```python
from build123d import *

# Parameters (mm, degrees)
BOSS_EXTRUDE1_DEPTH = 10


with BuildPart() as part:
    # Sketch1 → Boss-Extrude1 (new body)
    with BuildSketch(Plane.XY):
        with BuildLine():
            Line((138.578606851, 12), (138.578606851, 0))
            Line((138.578606851, 0), (37.275, 0))
            Line((37.275, 0), (37.275, 12))
            Line((37.275, 12), (38.178606851, 12))
            ThreePointArc((38.178606851, 12), (39.211044436, 12.32552632), (39.870053568, 13.184363742))
            Line((39.870053568, 13.184363742), (44.171321406, 25.002))
            Line((44.171321406, 25.002), (49.228678594, 25.002))
            Line((49.228678594, 25.002), (53.529946432, 13.184363742))
            ThreePointArc((53.529946432, 13.184363742), (54.188955564, 12.32552632), (55.221393149, 12))
            Line((55.221393149, 12), (57.028606851, 12))
            ThreePointArc((57.028606851, 12), (58.061044436, 12.32552632), (58.720053568, 13.184363742))
            Line((58.720053568, 13.184363742), (63.021321406, 25.002))
            Line((63.021321406, 25.002), (68.078678594, 25.002))
            Line((68.078678594, 25.002), (72.379946432, 13.184363742))
            ThreePointArc((72.379946432, 13.184363742), (73.038955564, 12.32552632), (74.071393149, 12))
            Line((74.071393149, 12), (75.878606851, 12))
            ThreePointArc((75.878606851, 12), (76.911044436, 12.32552632), (77.570053568, 13.184363742))
            Line((77.570053568, 13.184363742), (81.871321406, 25.002))
            Line((81.871321406, 25.002), (86.928678594, 25.002))
            Line((86.928678594, 25.002), (91.229946432, 13.184363742))
            ThreePointArc((91.229946432, 13.184363742), (91.888955564, 12.32552632), (92.921393149, 12))
            Line((92.921393149, 12), (94.728606851, 12))
            ThreePointArc((94.728606851, 12), (95.761044436, 12.32552632), (96.420053568, 13.184363742))
            Line((96.420053568, 13.184363742), (100.721321406, 25.002))
            Line((100.721321406, 25.002), (105.778678594, 25.002))
            Line((105.778678594, 25.002), (110.079946432, 13.184363742))
            ThreePointArc((110.079946432, 13.184363742), (110.738955564, 12.32552632), (111.771393149, 12))
            Line((111.771393149, 12), (113.578606851, 12))
            Line((113.578606851, 12), (138.578606851, 12))
        make_face()
    extrude(amount=BOSS_EXTRUDE1_DEPTH)


solid = part.part
```
The listing builds one solid part. Answer for the finished solid, in the listing's coordinates (mm). A direction names the side the tool comes from. Coordinates: 2 decimals unless noted, no trailing zeros. Write each loop counter-clockwise with the first axis right and the second up, starting at its lowest first coordinate (ties: lowest second). Pieces come first, ordered by that corner, then holes.
Q1. Section C-C, the plane x = 131 is taken. Write down the section's boundary in (y, z), then the cut area to 3 significant figures.
Returned:
outline: (0, 0) - (12, 0) - (12, 10) - (0, 10) - close
area: 120 mm2
Q2. Given P1, Ø0.5, axis at x = 37.5, z = 6.5, coming from the +Y side; P2, Ø2, axis at x = 56.5, z = 4.5, coming from the +Y side; P3, Ø1.5, axis at x = 108.5, y = 16, coming from the -Z side, each flat-ended and moving along its own axis, determine where each tip first touches the part or whether it passes through.
Returned:
P1: stops at y = 12
P2: stops at y = 12.06
P3: stops at z = 0
Q3. Which of the six approach directions +Z, -Z, +X, -X, +Y, -Y give full straight-line access (tool end or side, diameter ignored) to faces 1 (the cylindrical face through (54.18, 12.33, 4.93)), 2 (the flat face through (41.99, 19.01, 4.93)), 3 (the flat face through (125, 12, 5))?
Returned:
face 1: +Z, -Z, +Y
face 2: +Z, -Z, -X, +Y
face 3: +Z, -Z, +X, +Y
Q4. Section B-B, the plane y = 19 is taken. Write down the section's boundary in (x, z).
Returned:
outline: (41.99, 0) - (51.41, 0) - (51.41, 10) - (41.99, 10) - close; (60.84, 0) - (70.26, 0) - (70.26, 10) - (60.84, 10) - close; (79.69, 0) - (89.11, 0) - (89.11, 10) - (79.69, 10) - close; (98.54, 0) - (107.96, 0) - (107.96, 10) - (98.54, 10) - close
Q5. The mould has two halves that part along X. Classify faces 4 (the cylindrical face through (76.9, 12.32, 4.93)), 5 (the flat face through (37.275, 6, 5)), 6 (the flat face through (107.899, 19.176, 4.93)), 7 (the flat face through (103, 25.002, 5)): released by +X, released by -X, zero draft, split by the parting line, or undercut.
Returned:
face 4: undercut
face 5: released by -X
face 6: released by +X
face 7: zero draft
Q6. Section D-D, the plane x = 107.5 is taken. Write down the section's boundary in (y, z), then the cut area to 3 significant figures.
Returned:
outline: (0, 0) - (20.27, 0) - (20.27, 10) - (0, 10) - close
area: 203 mm2
Q7. Find the intervals of material crossed by line 1 along X through (y, z) = (23.25, 3.5); line 2 along X through (y, z) = (20, 0.75); line 3 along Y through (x, z) = (120.5, 9), in increasing order.
Returned:
line 1: x = 43.53 to 49.87, 62.38 to 68.72, 81.23 to 87.57, 100.08 to 106.42
line 2: x = 42.35 to 51.05, 61.2 to 69.9, 80.05 to 88.75, 98.9 to 107.6
line 3: y = 0 to 12
Q8. Section A-A, the plane z = 2.5 is taken. Write down the section's boundary in (x, y) (3 decimals).
Returned:
outline: (37.275, 0) - (138.579, 0) - (138.579, 12) - (111.771, 12) arc R1.8 cw to (110.08, 13.184) - (105.779, 25.002) - (100.721, 25.002) - (96.42, 13.184) arc R1.8 cw to (94.729, 12) - (92.921, 12) arc R1.8 cw to (91.23, 13.184) - (86.929, 25.002) - (81.871, 25.002) - (77.57, 13.184) arc R1.8 cw to (75.879, 12) - (74.071, 12) arc R1.8 cw to (72.38, 13.184) - (68.079, 25.002) - (63.021, 25.002) - (58.72, 13.184) arc R1.8 cw to (57.029, 12) - (55.221, 12) arc R1.8 cw to (53.53, 13.184) - (49.229, 25.002) - (44.171, 25.002) - (39.87, 13.184) arc R1.8 cw to (38.179, 12) - (37.275, 12) - close
